Autodesk Inventor part; units mm, degrees
ref_plane "YZ Plane" through (0, 0, 0) normal (1, 0, 0) x (0, 1, 0)
ref_plane "XZ Plane" through (0, 0, 0) normal (0, 1, 0) x (-1, 0, 0)
ref_plane "XY Plane" through (0, 0, 0) normal (0, 0, 1) x (1, 0, 0)
sketch "Sketch1" plane through (0, 0, 0) normal (0, 1, 0) x (-1, 0, 0)
  circle A0 centre (0, 0) radius 21.5
  circle A1 centre (0, 0) radius 55
  dimension "d0" = 43
  dimension "d1" = 110
extrude "Extrusion1" add sketch "Sketch1" along normal blind 20
sketch "Sketch2" plane through (0, 0, 0) normal (0, 0, 1) x (1, 0, 0)
  line L0 (0, 0) -> (0, 20)
  line L1 (55, 20) -> (-55, 20)
  circle A0 centre (-36.5, 17) radius 5
  line L2 (-21.5, 0) -> (-21.5, 20) construction
  line L3 (-21.5, 20) -> (-21.5, 0) construction
  dimension "d4" = 10
  dimension "d5" = 15
revolve "Revolution1" cut sketch "Sketch2" angle 360 about axis through (0, 0, 0) along (0, 1, 0)
sketch "Sketch3" plane through (0, 20, 0) normal (0, 1, 0) x (1, 0, 0)
  circle A0 centre (0, 0) radius 21.5
  circle A1 centre (0, 0) radius 26.5
  circle A2 centre (0, 0) radius 21.5
  dimension "d18" = 43
  dimension "d19" = 43
  dimension "d20" = 53
extrude "Extrusion2" add sketch "Sketch3" along normal blind 60
sketch "Sketch4" plane through (0, 0, 0) normal (1, 0, 0) x (0, 1, 0)
  line L0 (80, 21.5) -> (80, -21.5)
  line L1 (80, -21.5) -> (76, -19)
  line L2 (76, -19) -> (76, -21.5)
  line L3 (0, -21.5) -> (80, -21.5)
  line L4 (80, -21.5) -> (76, -21.5)
  line L5 (80, 0) -> (74, 0)
  point P0 (0, 0)
  dimension "d9" = 2.5
revolve "Revolution2" add sketch "Sketch4" angle 360 about axis through (0, 80, 0) along (0, -1, 0)
sketch "Sketch5" plane through (0, 80, 0) normal (0, 1, 0) x (1, 0, 0)
  line L0 (0, 4) -> (0, -4)
  line L1 (0, 0) -> (6.4984, 17.8542) construction
  line L2 (0, 0) -> (-6.4984, 17.8542) construction
  line L3 (0, 0) -> (9.0635, 24.9019) construction
  line L4 (0, 0) -> (0, 0) construction
  circle A0 centre (0, 0) radius 26.5
  arc A1 (-9.0635, 24.9019) -> (-9.0635, -24.9019) centre (0, 0) ccw
  line L5 (0, 0) -> (-9.0635, -24.9019) construction
  line L6 (0, 0) -> (-9.0635, 24.9019) construction
  arc A2 (9.0635, -24.9019) -> (9.0635, 24.9019) centre (0, 0) ccw
  line L7 (0, 0) -> (9.0635, -24.9019) construction
  line L8 (0, 0) -> (9.0635, 24.9019) construction
  circle A3 centre (0, 0) radius 19
  arc A4 (-6.4984, 17.8542) -> (-6.4984, -17.8542) centre (0, 0) ccw
  arc A5 (6.4984, -17.8542) -> (6.4984, 17.8542) centre (0, 0) ccw
  line L9 (-9.0635, -24.9019) -> (-6.4984, -17.8542)
  line L10 (6.4984, -17.8542) -> (9.0635, -24.9019)
  line L11 (6.4984, 17.8542) -> (9.0635, 24.9019)
  line L12 (-6.4984, 17.8542) -> (-9.0635, 24.9019)
  dimension "d22" = 40
  dimension "d23" = 40
  dimension "d24" = 20
  dimension "d25" = 20
  dimension "d26" = 140
  dimension "d27" = 140
extrude "Extrusion3" cut sketch "Sketch5" against normal blind 19 contours A0 L10 A3 L11 | L12 A3 L9 A0
sketch "Sketch6" plane through (0, 0, 0) normal (0, -1, 0) x (1, 0, 0)
  circle A0 centre (49, 0) radius 2
  circle A1 centre (-24.5, 42.4352) radius 2
  circle A2 centre (-24.5, -42.4352) radius 2
  point P0 (0, 0)
  dimension "d32" = 360
extrude "Extrusion4" cut sketch "Sketch6" against normal up to surface (20 mm away)
chamfer "Chamfer2" distance 2 angle 45 3 edges at (-26.5, 20, -42.4352) (-26.5, 20, 42.4352) (47, 20, 0)
equation "\"d19\" = d18"
properties part number "Blower Attachement"
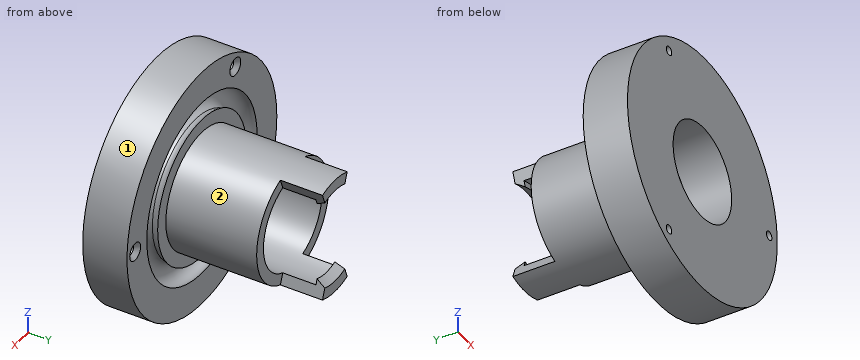
Input: part model. Units: mm. Frame: model coordinates. Face numbers are marked on the shaded views. A direction names the side the tool comes from. Give positions to 0.01 mm unless a question says otherwise; leave off trailing zeros. Order: outer loops, then holes, each group sorted by start corner. A loop starts at its lowest first (then second) coordinate and runs counter-clockwise, first axis right, second up.
1. Pin query (flat end, axial travel): pin 1 (1.8 mm diameter, centred on x = 0.5, z = 19.5, fed in from -Y); pin 2 (8 mm diameter, centred on y = 62, z = 10.5, fed in from +X); pin 3 (1 mm diameter, centred on y = 28, z = 3, fed in from +X). Return the tip coordinate at first contact, or that it passes through.
Derived:
pin 1: stops at y = 76
pin 2: stops at x = 25.66
pin 3: stops at x = 26.38
2. Section D-D on x = -24.5. Give the number of separate pieces and of enclosed holes in the cut face, and give its area (3 significant figures).
Derived:
separate pieces: 3
enclosed holes: 0
area: 2,450 mm2
3. Section C-C on y = 55. Return the cut outline in (x, z), and give its area (3 significant figures).
Derived:
outline: circle Ø53 at (0, 0); hole circle Ø43 at (0, 0)
area: 754 mm2
4. Reachability of the marked faces 1 and 2 from +Z, -Z, +X, -X, +Y, -Y: full face, straight path, thin tool, end or side. Return the list, or none.
Derived:
face 1: +Y, -Y
face 2: +Y
5. Section A-A on z = 0. Return the cut outline in (x, y).
Derived:
outline: (-55, 0) - (-21.5, 0) - (-21.5, 61) - (-26.5, 61) - (-26.5, 20) - (-32.5, 20) arc R5 cw (long way) to (-40.5, 20) - (-55, 20) - close; (21.5, 0) - (47, 0) - (47, 18) - (45, 20) - (40.5, 20) arc R5 cw (long way) to (32.5, 20) - (26.5, 20) - (26.5, 61) - (21.5, 61) - close; (51, 0) - (55, 0) - (55, 20) - (53, 20) - (51, 18) - close
6. Section B-B on x = 49. Return the cut outline in (y, z), and give its area (3 significant figures).
Derived:
outline: (0, -24.98) - (20, -24.98) - (20, -4) - (18, -2) - (0, -2) - close; (0, 2) - (18, 2) - (20, 4) - (20, 24.98) - (0, 24.98) - close
area: 915 mm2
7. Material intervals for L1, parallel to Z at x = 0, y = 51; L2, parallel to Z at x = 0, y = 6; L3, parallel to Z at x = 0, y = 13, sorted ascending.
Derived:
L1: z = -26.5 to -21.5, 21.5 to 26.5
L2: z = -55 to -21.5, 21.5 to 55
L3: z = -55 to -39.5, -33.5 to -21.5, 21.5 to 33.5, 39.5 to 55
